The listing builds one solid part. Answer for the finished solid, in the listing's coordinates (mm). Face numbers are marked on the shaded views. Coordinates: 2 decimals unless noted, no trailing zeros. Order: outer loops, then holes, each group sorted by start corner. A loop starts at its lowest first (then second) coordinate and runs counter-clockwise, first axis right, second up. Notation, with made-up numbers: (41, 74.5) - (62, 74.5) arc R7 cw to (62, 86.5) - close; hole circle Ø8 at (19.5, 76). An arc over 180 degrees is marked (long way). Use one line per item in the form item = value. Start each with the question number.
Item 1: Section C-C, the plane z = 24 is taken. Write down the section's boundary in (x, y).
Item 2: Section A-A, the plane y = 0 is taken. Write down the section's boundary in (x, z).
Item 3: Consider line 1 along Y through (x, z) = (0, 6.6); line 2 along Y through (x, z) = (0, 25.25); line 3 along X through (y, z) = (2.25, 13.75). Determine where each line is inside the solid, lowest interval first. Write a range as [from, to].
Item 4: Each of these flat-tipped pins is pushed along its axis until it touches: pin 1 Ø4.5 at (x, y) = (0, 0) entering from +Z; pin 2 Ø5 at (x, y) = (2, -1.5) entering from +Z. Where does it stop, or does it pass through?
Item 5: Section B-B, the plane x = 0 is taken. Write down the section's boundary in (y, z), and give its area (3 significant figures).
Item 6: The mould has two halves that part along Y. Classify the marked faces 1, 2, 3 and 4: released by +Y, released by -Y, zero draft, split by the parting line, or undercut.
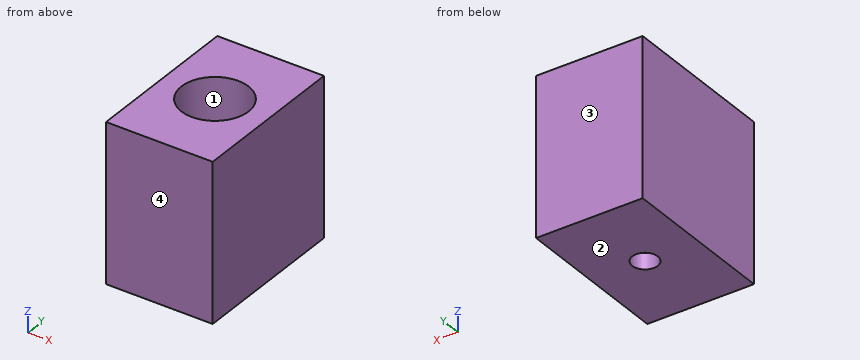
from build123d import *

# Parameters (mm, degrees)
F2_W     = 20
F2_H     = 30
F2_R     = 8.3
F3_DEPTH = 29.6


with BuildPart() as f1:
    # F0 (on Front) → F1 (revolve)
    with BuildSketch(Plane.XZ):
        Polygon((-3.6, 3), (-3.6, 3.4), (-5.9, 5.6), (-5.9, 9.6), (-6.3, 10.6), (-6.3, 29.6), (-8.3, 29.6), (-8.3, 0), (-2.4, 0), (-2.4, 3), align=None)
    revolve(axis=Axis((0, 0, 14.8), (0, 0, -1)))

    # F2 (on face) → F3 (join)
    with BuildSketch(Plane(origin=(0, 0, 0), x_dir=(1, 0, 0), z_dir=(0, 0, -1))):
        Rectangle(F2_W, F2_H)
        Circle(F2_R, mode=Mode.SUBTRACT)
    extrude(amount=-F3_DEPTH)


solid = f1.part
Response:
q1.outline = (-10, -15) - (10, -15) - (10, 15) - (-10, 15) - close; hole circle Ø12.6 at (0, 0)
q2.outline = (-10, 0) - (-2.4, 0) - (-2.4, 3) - (-3.6, 3) - (-3.6, 3.4) - (-5.9, 5.6) - (-5.9, 9.6) - (-6.3, 10.6) - (-6.3, 29.6) - (-10, 29.6) - close; (2.4, 0) - (10, 0) - (10, 29.6) - (6.3, 29.6) - (6.3, 10.6) - (5.9, 9.6) - (5.9, 5.6) - (3.6, 3.4) - (3.6, 3) - (2.4, 3) - close
q3.line_1 = [-15, -5.9], [5.9, 15]
q3.line_2 = [-15, -6.3], [6.3, 15]
q3.line_3 = [-10, -5.88], [5.88, 10]
q4.pin_1 = through
q4.pin_2 = 4.74
q5.outline = (-15, 0) - (-2.4, 0) - (-2.4, 3) - (-3.6, 3) - (-3.6, 3.4) - (-5.9, 5.6) - (-5.9, 9.6) - (-6.3, 10.6) - (-6.3, 29.6) - (-15, 29.6) - close; (2.4, 0) - (15, 0) - (15, 29.6) - (6.3, 29.6) - (6.3, 10.6) - (5.9, 9.6) - (5.9, 5.6) - (3.6, 3.4) - (3.6, 3) - (2.4, 3) - close
q5.area = 551 mm2
q6.face_1 = undercut
q6.face_2 = zero draft
q6.face_3 = released by +Y
q6.face_4 = released by -Y
